The model under review builds one solid part; all positions refer to its coordinate system, in mm. A direction names the side the tool comes from. Coordinates: 2 decimals unless noted, no trailing zeros. Order: outer loops, then holes, each group sorted by start corner. A loop starts at its lowest first (then second) coordinate and runs counter-clockwise, first axis right, second up. Notation, with made-up numbers: (71, 34) -> (100, 34) arc R18 cw to (100, 49) -> close; hole circle Ø4 at (-15, -20). An arc over 180 degrees is marked (long way). Put each result on its own line as item: value.
from build123d import *

# Parameters (mm, degrees)
SKETCH1_W                       = 140
SKETCH1_H                       = 40
SKETCH1_W_2                     = 6.3
SKETCH1_H_2                     = 6.3
BOSS_EXTRUDE1_DEPTH             = 12.7
TAP_DRILL_FOR_M4X0_7_TAP1_D     = 3.3
TAP_DRILL_FOR_M4X0_7_TAP1_DEPTH = 12.1
TAP_DRILL_FOR_M5X0_8_TAP2_D     = 4.2
TAP_DRILL_FOR_M5X0_8_TAP2_DEPTH = 7
TAP_DRILL_FOR_M5X0_8_TAP2_TIP   = 1.2618073


with BuildPart() as part:
    # Sketch1 → Boss-Extrude1 (new body)
    with BuildSketch(Plane.XY):
        with Locations((0, 20)):
            Rectangle(SKETCH1_W, SKETCH1_H)
        with Locations((35, 24.75)):
            Rectangle(SKETCH1_W_2, SKETCH1_H_2, mode=Mode.SUBTRACT)
    extrude(amount=BOSS_EXTRUDE1_DEPTH)

    # Tap Drill for M4x0.7 Tap1
    with Locations(Plane(origin=(35, 40, 6.35), x_dir=(0, 0, 1), z_dir=(0, 1, 0))):
        with Locations((0, 0)):
            Hole(TAP_DRILL_FOR_M4X0_7_TAP1_D / 2, depth=TAP_DRILL_FOR_M4X0_7_TAP1_DEPTH)

    # Tap Drill for M5x0.8 Tap2
    with Locations(Plane(origin=(-60, 0, 6.35), x_dir=(0, 0, -1), z_dir=(0, -1, 0))):
        with Locations((0, 0), (0, 60), (0, 120)):
            Hole(TAP_DRILL_FOR_M5X0_8_TAP2_D / 2, depth=TAP_DRILL_FOR_M5X0_8_TAP2_DEPTH)
            with Locations((0, 0, -(TAP_DRILL_FOR_M5X0_8_TAP2_DEPTH + TAP_DRILL_FOR_M5X0_8_TAP2_TIP / 2))):  # 118° drill point
                Cone(0, TAP_DRILL_FOR_M5X0_8_TAP2_D / 2, TAP_DRILL_FOR_M5X0_8_TAP2_TIP, mode=Mode.SUBTRACT)


solid = part.part
Item 1: Consider section A-A on y = 26.5. Write out the cut boundary in (x, z), and give its area (3 significant figures).
Answers below:
outline: (-70, 0) -> (31.85, 0) -> (31.85, 12.7) -> (-70, 12.7) -> close; (38.15, 0) -> (70, 0) -> (70, 12.7) -> (38.15, 12.7) -> close
area: 1,700 mm^2
Item 2: Mouldability with a two-part tool opening along Y and no side actions: class faces 1 (the flat face through (-1, 0, 9)), 2 (the flat face through (70, 20, 6)), 3 (the flat face through (38.15, 25, 6)) as +Y half, -Y half, draft (parallel to the pull), parting line (faces both ways), or undercut.
Answers below:
face 1: -Y half
face 2: draft
face 3: undercut
Item 3: For line 1 (X direction, y = 2.25, z = 6.35); line 2 (Z direction, x = -60, y = 1.75); line 3 (X direction, y = 34.25, z = 6.35), list the stretches that pass through material, from the lowest coordinate up. Write a range as from..to.
Answers below:
line 1: -70..-62.1, -57.9..-2.1, 2.1..57.9, 62.1..70
line 2: 0..4.25, 8.45..12.7
line 3: -70..33.35, 36.65..70
Item 4: For faces 4 (the cylindrical face through (57.95, 3.55, 5.89)), 5 (the flat face through (31.85, 25, 6)), 6 (the cylindrical face through (36.39, 33.87, 5.46)), 7 (the flat face through (-70, 20, 6)), list the 3-axis set-ups (+Z, -Z, +X, -X, +Y, -Y) from which the entire face can be reached by the end or side of a thin tool; tool diameter is ignored.
Answers below:
face 4: -Y
face 5: +Z, -Z
face 6: +Y
face 7: +Z, -Z, -X, +Y, -Y
